CAD build for the part. Positions are in the model's coordinates, mm. Face numbers are marked on the shaded views. Give positions to 0.01 mm unless a question says otherwise; leave off trailing zeros. Loops run counter-clockwise (first coordinate to the right, second up) from the corner with the lowest first, then second, coordinate; pieces in that order, holes last.
Item 1: Probe probe 1 along Z at (x, y) = (0, -9); probe 2 along Z at (x, y) = (-31.5, -22); probe 3 along X at (y, z) = (-13.5, -52). List the from-to ranges inside material, lowest first.
Item 2: Drop flat-ended pins along their axis: P1, Ø1, axis at x = -11, z = 14.5, coming from the +Y side; P2, Ø4, axis at y = -7, z = 5, coming from the -X side; P3, Ø12, axis at y = -3, z = -35.5, coming from the -X side; P4, Ø12, axis at y = -6.5, z = 36, coming from the +X side. Give the stop position or say it passes through.
Item 3: Saw through at C-C on y = -9.75. Give the cut face in (x, z).
Item 4: Saw through at B-B on x = 0. Give the cut face in (y, z), plus the area to 3 significant figures.
Item 5: Saw through at D-D on x = 49. Give the cut face in (y, z).
Item 6: Saw through at A-A on z = 0. Give the cut face in (x, y).
Item 7: Mould opens along X. For the marked faces 1, 2, 3 and 4 say: released by +X, released by -X, zero draft, split by the parting line, or undercut.
from build123d import *

# Parameters (mm, degrees)
F0_R     = 8.5
F0_R_2   = 19
F1_DEPTH = 25


with BuildPart() as f1:
    # F0 (on Front) → F1 (new body)
    with BuildSketch(Plane.XZ):
        with BuildLine():
            Line((-43.715996, 59.483897), (-58.76085, 29.010438))
            ThreePointArc((-58.76085, 29.010438), (-65.532, 0), (-58.76085, -29.010438))
            Line((-58.76085, -29.010438), (-43.715996, -59.483897))
            ThreePointArc((-43.715996, -59.483897), (-38.470598, -65.267388), (-30.9626, -67.4105))
            Line((-30.9626, -67.4105), (30.9626, -67.4105))
            ThreePointArc((30.9626, -67.4105), (38.470598, -65.267388), (43.715996, -59.483897))
            Line((43.715996, -59.483897), (58.76085, -29.010438))
            ThreePointArc((58.76085, -29.010438), (65.532, 0), (58.76085, 29.010438))
            Line((58.76085, 29.010438), (43.715996, 59.483897))
            ThreePointArc((43.715996, 59.483897), (38.470598, 65.267388), (30.9626, 67.4105))
            Line((30.9626, 67.4105), (-30.9626, 67.4105))
            ThreePointArc((-30.9626, 67.4105), (-38.470598, 65.267388), (-43.715996, 59.483897))
        make_face()
        with Locations((-30.9626, -53.1875)):
            Circle(F0_R, mode=Mode.SUBTRACT)
        with Locations((30.9626, -53.1875)):
            Circle(F0_R, mode=Mode.SUBTRACT)
        Circle(F0_R_2, mode=Mode.SUBTRACT)
        with Locations((-30.9626, 53.1875)):
            Circle(F0_R, mode=Mode.SUBTRACT)
        with Locations((30.9626, 53.1875)):
            Circle(F0_R, mode=Mode.SUBTRACT)
    extrude(amount=F1_DEPTH)


solid = f1.part
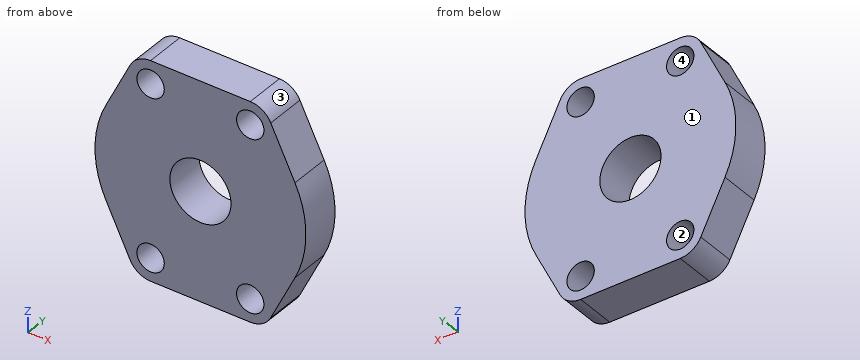
Results below:
1. probe 1: z = -67.41 to -19, 19 to 67.41
1. probe 2: z = -67.4 to -61.67, -44.7 to 44.7, 61.67 to 67.4
1. probe 3: x = -47.41 to -39.38, -22.55 to 22.55, 39.38 to 47.41
2. P1: passes through
2. P2: stops at x = -65.46
2. P3: stops at x = -58.52
2. P4: stops at x = 58.27
3. outline: (-58.76, -29.01) - (-43.72, -59.48) arc R14.22 ccw to (-30.96, -67.41) - (30.96, -67.41) arc R14.22 ccw to (43.72, -59.48) - (58.76, -29.01) arc R65.53 ccw to (58.76, 29.01) - (43.72, 59.48) arc R14.22 ccw to (30.96, 67.41) - (-30.96, 67.41) arc R14.22 ccw to (-43.72, 59.48) - (-58.76, 29.01) arc R65.53 ccw to start; hole circle Ø17 at (-30.96, -53.19); hole circle Ø17 at (-30.96, 53.19); hole circle Ø38 at (0, 0); hole circle Ø17 at (30.96, -53.19); hole circle Ø17 at (30.96, 53.19)
4. outline: (-25, -67.41) - (0, -67.41) - (0, -19) - (-25, -19) - close; (-25, 19) - (0, 19) - (0, 67.41) - (-25, 67.41) - close
4. area: 2,420 mm2
5. outline: (-25, -48.78) - (0, -48.78) - (0, 48.78) - (-25, 48.78) - close
6. outline: (-65.53, -25) - (-19, -25) - (-19, 0) - (-65.53, 0) - close; (19, -25) - (65.53, -25) - (65.53, 0) - (19, 0) - close
7. face 1: zero draft
7. face 2: undercut
7. face 3: released by +X
7. face 4: undercut
